from build123d import *

# Parameters (mm, degrees)
SKETCH2_R                 = 14.2875
BOSS_EXTRUDE1_DEPTH       = 4.7625
TAP_DRILL_FOR_8_32_TAP1_D = 3.4544
F_10_CLEARANCE_HOLE1_D    = 4.9784


with BuildPart() as part:
    # Sketch2 → Boss-Extrude1 (new body)
    with BuildSketch(Plane(origin=(0, 0, 0), x_dir=(1, 0, 0), z_dir=(0, 1, 0))):
        with BuildLine():
            Line((19.05, 0), (-19.05, 0))
            Line((-19.05, 0), (-19.05, -26.9875))
            Line((-19.05, -26.9875), (-48.883968147, -39.985679272))
            ThreePointArc((-48.883968147, -39.985679272), (-58.667673568, -65.221680031), (-33.341491014, -74.769512421))
            Line((-33.341491014, -74.769512421), (19.05, -50.8))
            Line((19.05, -50.8), (19.05, 0))
        make_face()
        with Locations(Location((-41.275, -57.450103217, 0), (0, 0, 90))):
            Circle(SKETCH2_R, mode=Mode.SUBTRACT)
    extrude(amount=BOSS_EXTRUDE1_DEPTH)

    # Tap Drill for #8-32 Tap1 (through all)
    with Locations(Plane(origin=(0, 4.7625, 0), x_dir=(1, 0, 0), z_dir=(0, 1, 0))):
        with Locations((-24.742011998, -50.246946705)):
            Hole(TAP_DRILL_FOR_8_32_TAP1_D / 2)

    # #10 Clearance Hole1 (through all)
    with Locations(Plane(origin=(0, 4.7625, 0), x_dir=(1, 0, 0), z_dir=(0, 1, 0))):
        with Locations((-12.7, -19.05), (12.7, -19.05)):
            Hole(F_10_CLEARANCE_HOLE1_D / 2)


solid = part.part
Check sheet for the modelled part. Datum: model origin and axes. Units: mm. A direction names the side the tool comes from. Coordinates: 2 decimals unless noted, no trailing zeros. Loops run counter-clockwise (first coordinate to the right, second up) from the corner with the lowest first, then second, coordinate; pieces in that order, holes last. Notation, with made-up numbers: (-22.5, 68) -> (14.5, 68) arc R21 cw to (14.5, 73) -> close; hole circle Ø8 at (65, -26.5). An arc over 180 degrees is marked (long way). Answer in a Markdown table with one row per item.
1. Sectioned sample at A-A, the plane z = 19.05. Record the boundary of the cut face in (x, y), then the cut area to 3 significant figures.
Check values:
| item | result |
|---|---|
| outline | (-19.05, 0) -> (-15.19, 0) -> (-15.19, 4.76) -> (-19.05, 4.76) -> close; (-10.21, 0) -> (10.21, 0) -> (10.21, 4.76) -> (-10.21, 4.76) -> close; (15.19, 0) -> (19.05, 0) -> (19.05, 4.76) -> (15.19, 4.76) -> close |
| area | 134 mm2 |
2. Sectioned sample at D-D, the plane z = 46. Record the boundary of the cut face in (x, y), then the cut area to 3 significant figures.
Check values:
| item | result |
|---|---|
| outline | (-56.5, 0) -> (-49.82, 0) -> (-49.82, 4.76) -> (-56.5, 4.76) -> close; (-32.73, 0) -> (19.05, 0) -> (19.05, 4.76) -> (-32.73, 4.76) -> close |
| area | 278 mm2 |
3. Material ranges on line 1 along X through (y, z) = (1.4, 19.05); line 2 along X through (y, z) = (1.1, 50); line 3 along X through (y, z) = (3.75, 5), recorded low to high. Write a range as [from, to].
Check values:
| item | result |
|---|---|
| line 1 | x = [-19.05, -15.19], [-10.21, 10.21], [15.19, 19.05] |
| line 2 | x = [-58.81, -53.47], [-29.08, -26.45], [-23.03, 19.05] |
| line 3 | x = [-19.05, 19.05] |
4. Release check for a two-part mould opening along X. For faces 1 (the face through (0, 2, 0)), 2 (the face through (-33.758, 2.348, 33.396)), 3 (the face through (-35.803, 2.348, 44.252)) record: released by +X, released by -X, zero draft, split by the parting line, or undercut.
Check values:
| item | result |
|---|---|
| face 1 | zero draft |
| face 2 | released by -X |
| face 3 | undercut |
5. Sectioned sample at B-B, the plane x = -37.5. Record the boundary of the cut face in (y, z), then the cut area to 3 significant figures.
Check values:
| item | result |
|---|---|
| outline | (0, 35.03) -> (4.76, 35.03) -> (4.76, 43.67) -> (0, 43.67) -> close; (0, 71.23) -> (4.76, 71.23) -> (4.76, 76.12) -> (0, 76.12) -> close |
| area | 64.5 mm2 |
6. Go/stop test with flat-tipped pins: pin 1 (1 mm diameter, centred on y = 2.5, z = 9, fed in from -X); pin 2 (4 mm diameter, centred on x = -12.7, z = 19.05, fed in from +Y); pin 3 (1.5 mm diameter, centred on y = 4, z = 44.5, fed in from -X); pin 4 (1 mm diameter, centred on y = 1, z = 28.5, fed in from -X). Record where each tip stops, or that it passes through.
Check values:
| item | result |
|---|---|
| pin 1 | stops at x = -19.05 |
| pin 2 | passes through |
| pin 3 | stops at x = -55.91 |
| pin 4 | stops at x = -23.67 |
7. Access from +Z, -Z, +X, -X, +Y, -Y to the whole of each face (thin tool, end or side, straight path). Record for faces 4 (the face through (-12, 0, 38)), 5 (the face through (-19.05, 2, 13)).
Check values:
| item | result |
|---|---|
| face 4 | +Z, -Z, +X, -X, -Y |
| face 5 | -Z, -X, +Y, -Y |
8. Sectioned sample at C-C, the plane y = 3.4. Give the number of separate pieces and of enclosed holes in the cut face, then the cut area to 3 significant figures.
Check values:
| item | result |
|---|---|
| separate pieces | 1 |
| enclosed holes | 4 |
| area | 3,070 mm2 |
